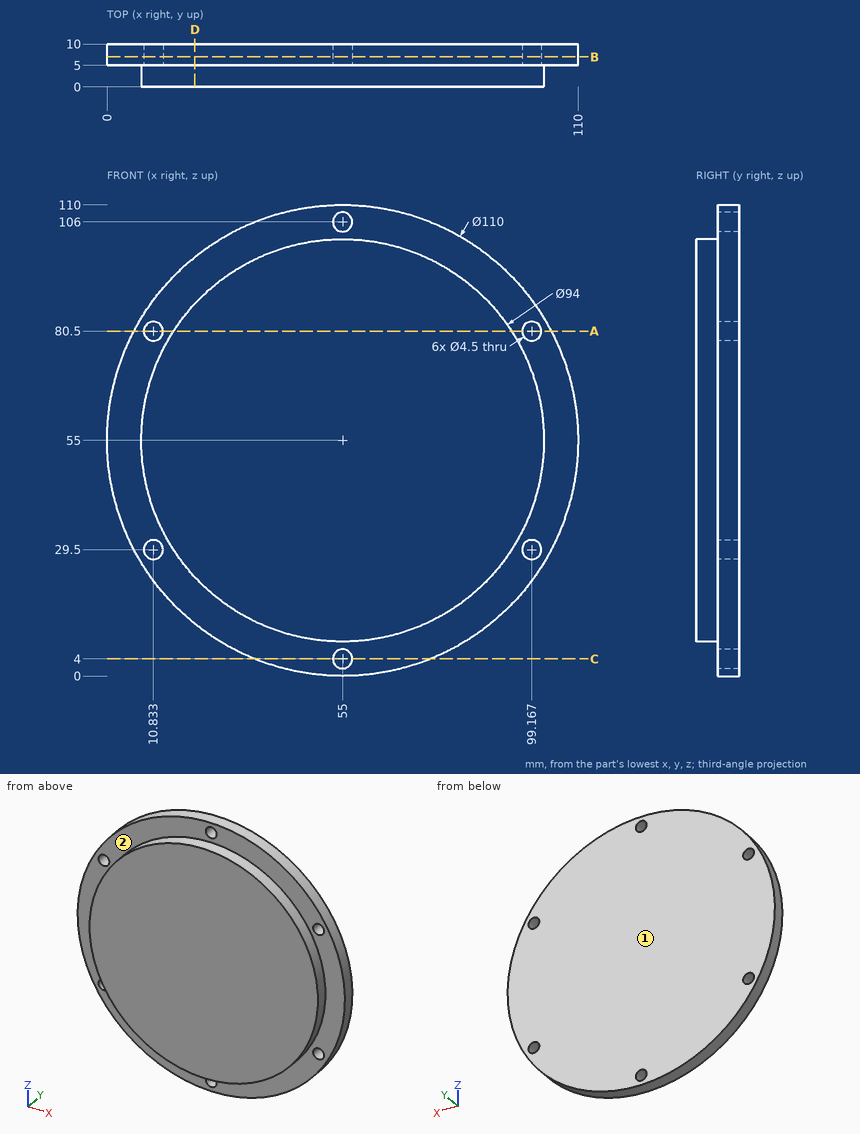
Answer from the drawing. Dimensions are ordinates in mm from the lowest x, y and z of the part. A direction names the side the tool comes from. Give positions to 0.01 mm unless a question says otherwise; leave off trailing zeros. Loops run counter-clockwise (first coordinate to the right, second up) from the corner with the lowest first, then second, coordinate; pieces in that order, holes last.
Item 1: The part is cut by section C-C (z = 4). Write down the section's boundary in (x, y), and give its area (3 significant figures).
Item 2: The part is cut by section A-A (z = 80.5). Write down the section's boundary in (x, y).
Item 3: Each of these flat-tipped pins is pushed along its axis until it touches: pin 1 Ø6 at (x, y) = (65, 8) entering from -Z; pin 2 Ø1.5 at (x, y) = (87, 5) entering from +Z; pin 3 Ø5 at (y, z) = (7.5, 84) entering from -X (1 decimal). Where does it stop, or does it pass through?
Item 4: The part is cut by section D-D (x = 20.5). Write down the section's boundary in (y, z).
Item 5: The part is cut by section B-B (y = 7). Write down the section's boundary in (x, z), and give its area (3 significant figures).
Item 6: Find the intervals of material crossed by line 1 along X through (y, z) = (7.75, 80.5); line 2 along X through (y, z) = (6.25, 81); line 3 along Y through (x, z) = (30.5, 10), in increasing order.
Item 7: For the marked faces 1 and 2, determine the directions among +Z, -Z, +X, -X, +Y, -Y from which every point of the face is accessible in a straight line to the end or side of a thin tool.
Taken from the geometry:
1. outline: (34.41, 5) - (52.75, 5) - (52.75, 10) - (34.41, 10) - close; (57.25, 5) - (75.59, 5) - (75.59, 10) - (57.25, 10) - close
1. area: 183 mm2
2. outline: (6.27, 5) - (8.58, 5) - (8.58, 10) - (6.27, 10) - close; (13.08, 5) - (15.52, 5) - (15.52, 0) - (94.48, 0) - (94.48, 5) - (96.92, 5) - (96.92, 10) - (13.08, 10) - close; (101.42, 5) - (103.73, 5) - (103.73, 10) - (101.42, 10) - close
3. pin 1: stops at z = 0.45
3. pin 2: stops at z = 100.26
3. pin 3: stops at x = 6.8
4. outline: (0, 23.08) - (5, 23.08) - (5, 12.17) - (10, 12.17) - (10, 97.83) - (5, 97.83) - (5, 86.92) - (0, 86.92) - close
5. outline: circle Ø110 at (55, 55); hole circle Ø4.5 at (10.83, 29.5); hole circle Ø4.5 at (10.83, 80.5); hole circle Ø4.5 at (55, 4); hole circle Ø4.5 at (55, 106); hole circle Ø4.5 at (99.17, 29.5); hole circle Ø4.5 at (99.17, 80.5)
5. area: 9,410 mm2
6. line 1: x = 6.27 to 8.58, 13.08 to 96.92, 101.42 to 103.73
6. line 2: x = 6.53 to 8.64, 13.03 to 96.97, 101.36 to 103.47
6. line 3: y = 5 to 10
7. face 1: +Z, -Z, +X, -X, +Y
7. face 2: -Y
